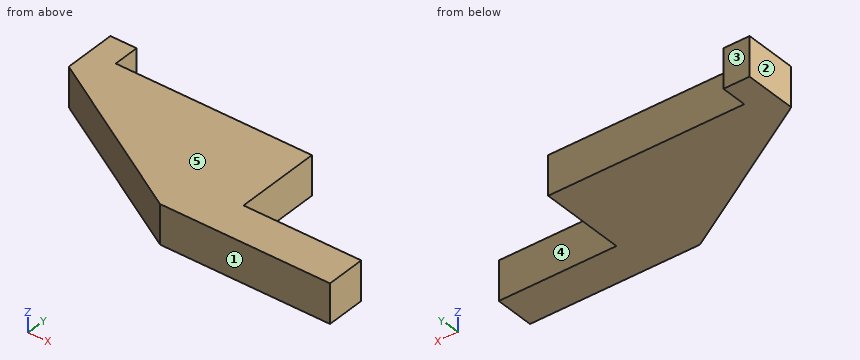
```python
from build123d import *

# Parameters (mm, degrees)
BOSS_EXTRUDE1_DEPTH      = 7.5
BOSS_EXTRUDE1_DEPTH_BACK = 7.5


with BuildPart() as part:
    # Sketch1 → Boss-Extrude1 (new, two sides: drawn at the far end of the back side and taken through both)
    with BuildSketch(Plane.XY.offset(-BOSS_EXTRUDE1_DEPTH_BACK)):
        Polygon((-451.871999052, -4.232779954), (-451.871999052, -19.232779954), (-516.871999052, -19.232779954), (-581.871999052, 18.567220046), (-581.871999052, 38.567220046), (-571.871999052, 38.567220046), (-571.871999052, 28.567220046), (-496.871999052, 28.567220046), (-496.871999052, -4.232779954), align=None)
    extrude(amount=BOSS_EXTRUDE1_DEPTH + BOSS_EXTRUDE1_DEPTH_BACK)


solid = part.part
```
Geometry check sheet. Reference: the model listing, model coordinates, mm. Face numbers are marked on the shaded views. A direction names the side the tool comes from. Coordinates: 2 decimals unless noted, no trailing zeros. Loops run counter-clockwise (first coordinate to the right, second up) from the corner with the lowest first, then second, coordinate; pieces in that order, holes last.
Item 1: Sectioned sample at C-C, the plane y = 31.5. Record the boundary of the cut face in (x, z).
Item 2: Access from +Z, -Z, +X, -X, +Y, -Y to the whole of each face (thin tool, end or side, straight path). Record for the marked faces 4 and 5.
Item 3: Thickness scan on line 1 (Y direction, x = -459, z = -4.25); line 2 (X direction, y = 21.5, z = 0.25); line 3 (Y direction, x = -513, z = -1.25). Record the ranges inside material, lowest first.
Item 4: Sectioned sample at A-A, the plane z = 2.5. Record the boundary of the cut face in (x, y).
Item 5: Release check for a two-part mould opening along Y. For the marked faces 1, 2 and 3 record: released by +Y, released by -Y, zero draft, split by the parting line, or undercut.
Item 6: Sectioned sample at B-B, the plane x = -503. Record the boundary of the cut face in (y, z).
Item 7: Go/stop test with flat-tipped pins: pin 1 Ø8 at (y, z) = (-4, -3) entering from -X; pin 2 Ø2 at (y, z) = (30, 4.5) entering from +X; pin 3 Ø2 at (x, z) = (-472.5, 1.5) entering from +Y. Record where each tip stops, or that it passes through.
Check result:
1. outline: (-581.87, -7.5) - (-571.87, -7.5) - (-571.87, 7.5) - (-581.87, 7.5) - close
2. face 4: +Z, -Z, +X, +Y
2. face 5: +Z, +X, -X, +Y, -Y
3. line 1: y = -19.23 to -4.23
3. line 2: x = -581.87 to -496.87
3. line 3: y = -19.23 to 28.57
4. outline: (-581.87, 18.57) - (-516.87, -19.23) - (-451.87, -19.23) - (-451.87, -4.23) - (-496.87, -4.23) - (-496.87, 28.57) - (-571.87, 28.57) - (-571.87, 38.57) - (-581.87, 38.57) - close
5. face 1: released by -Y
5. face 2: zero draft
5. face 3: released by +Y
6. outline: (-19.23, -7.5) - (28.57, -7.5) - (28.57, 7.5) - (-19.23, 7.5) - close
7. pin 1: stops at x = -549.94
7. pin 2: stops at x = -571.87
7. pin 3: stops at y = -4.23
